```python
from build123d import *


with BuildPart() as part:
    # Schizzo2 → Rivoluzione1 (revolve)
    with BuildSketch(Plane(origin=(0, 0, 0), x_dir=(0, 0, -1), z_dir=(1, 0, 0)), mode=Mode.PRIVATE) as rivoluzione1_sk:
        Polygon((0, 0), (0, 3), (6, 3), (6, 5), (8, 5), (8, 2.5), (13, 2.5), (15.7, 2.5), (15.7, 0), align=None)
    revolve(rivoluzione1_sk.sketch.rotate(Axis((0, 0, 0), (0, 0, -1)), 90), axis=Axis((0, 0, 0), (0, 0, -1)))


solid = part.part
```
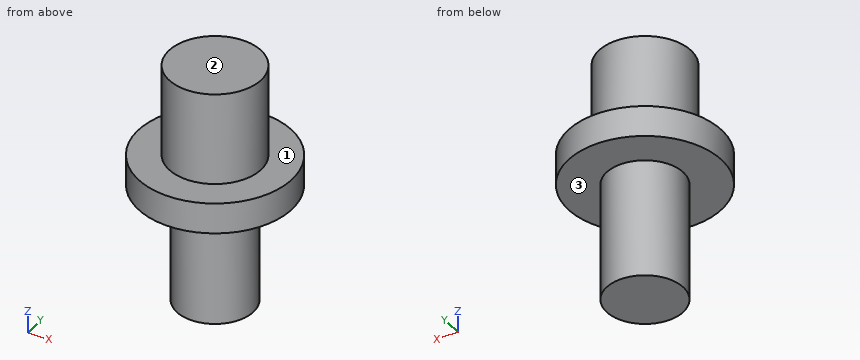
Build history of the part. All positions in model axes, mm. Face numbers are marked on the shaded views. A direction names the side the tool comes from. Round coordinates to 2 decimals unless told otherwise and drop trailing zeros. Loops run counter-clockwise (first coordinate to the right, second up) from the corner with the lowest first, then second, coordinate; pieces in that order, holes last.
Item 1: Which spindle directions (+Z, -Z, +X, -X, +Y, -Y) get a long thin tool onto all of the face, cutting with end or side? Do the marked faces 1, 2 and 3. Say none if no direction does.
Item 2: Drill centre lines: line 1 along Z through (x, y) = (-3.5, 0); line 2 along X through (y, z) = (-4, -7). Where is each one in solid material? Low to high.
Item 3: Pin check, flat tips, straight feed: P1, Ø2, axis at x = 3.5, y = 0.5, coming from the -Z side; P2, Ø1.5, axis at x = 2, z = -3, coming from the -Y side; P3, Ø1, axis at x = 2, z = -10.5, coming from the +Y side. Stop position of each tip, or through.
Item 4: Saw through at D-D (x = 2.75). List the corners of the cut face in (y, z), then the cut area to 3 significant figures.
Item 5: Saw through at A-A (x = 0). List the corners of the cut face in (y, z), then the cut area to 3 significant figures.
Item 6: Saw through at C-C (z = -5.5). List the corners of the cut face in (x, y), then the cut area to 3 significant figures.
Worked answers:
1. face 1: +Z
1. face 2: +Z, +X, -X, +Y, -Y
1. face 3: -Z
2. line 1: z = -8 to -6
2. line 2: x = -3 to 3
3. P1: stops at z = -8
3. P2: stops at y = -2.73
3. P3: stops at y = 2
4. outline: (-4.18, -8) - (4.18, -8) - (4.18, -6) - (1.2, -6) - (1.2, 0) - (-1.2, 0) - (-1.2, -6) - (-4.18, -6) - close
4. area: 31.1 mm2
5. outline: (-5, -8) - (-2.5, -8) - (-2.5, -15.7) - (2.5, -15.7) - (2.5, -8) - (5, -8) - (5, -6) - (3, -6) - (3, 0) - (-3, 0) - (-3, -6) - (-5, -6) - close
5. area: 94.5 mm2
6. outline: circle Ø6 at (0, 0)
6. area: 28.3 mm2
